The model under review builds one solid part; all positions refer to its coordinate system, in mm. Face numbers are marked on the shaded views. Round coordinates to 2 decimals unless told otherwise and drop trailing zeros. Loops run counter-clockwise (first coordinate to the right, second up) from the corner with the lowest first, then second, coordinate; pieces in that order, holes last. Notation, with made-up numbers: (-36.5, 14.25) -> (21.5, 14.25) arc R21 cw to (21.5, 42.25) -> close; hole circle Ø2 at (27.25, 41). An arc over 180 degrees is marked (long way). Write each question's results on one line, items separated by ' | '. Start each with the question number.
Item 1: We need section C-C (z = 2). Give the boundary of the cut face in (x, y), and give its area (3 significant figures).
Item 2: Mouldability with a two-part tool opening along X and no side actions: class the marked faces 1, 2 and 3 as pulls with the +X half, pulls with the -X half, needs draft (parallel to the pull), parting line crosses it, or undercut.
Item 3: Clearance check with flat-ended pins moving along their axes: pin 1 Ø4 at (x, z) = (52, 6) entering from +Y; pin 2 Ø5 at (y, z) = (24, 7) entering from +X; pin 3 Ø5 at (y, z) = (-45.5, 11.5) entering from -X; pin 4 Ø1 at (x, y) = (30, 16) entering from -Z. State where each tip first meets the part, or that it passes through.
Item 4: For L1, parallel to Y at x = 0, z = 3.5; L2, parallel to Z at x = 25.5, y = -18; L3, parallel to X at y = -19.5, z = 6.75, list the stretches that pass through material, from the lowest coordinate up. Write a range as from..to.
Item 5: We need section A-A (y = 0). Give the boundary of the cut face in (x, z).
Item 6: We need section D-D (y = 37.25). Give the boundary of the cut face in (x, z), and give its area (3 significant figures).
Item 7: We need section B-B (x = -72.5). Give the boundary of the cut face in (y, z), and give its area (3 significant figures).
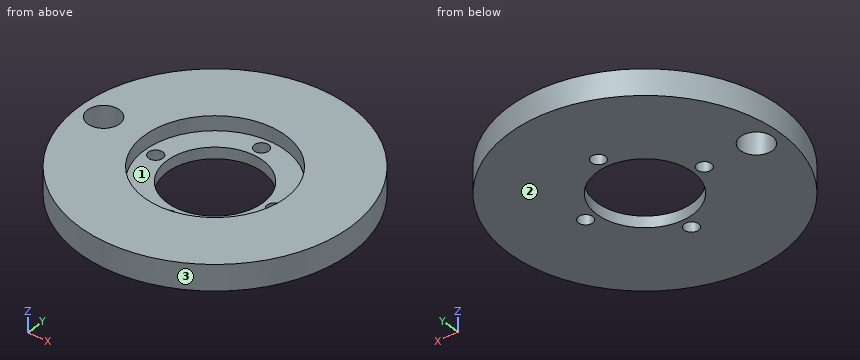
from build123d import *

# Parameters (mm, degrees)
F0_R     = 85
F0_R_2   = 4.5
F0_R_3   = 10
F0_R_4   = 30
F1_DEPTH = 16
F2_R     = 44.25
F2_R_2   = 4.5
F2_R_3   = 30
F3_DEPTH = 9


with BuildPart() as f1:
    # F0 (on Top) → F1 (new body)
    with BuildSketch(Plane.XY):
        Circle(F0_R)
        with Locations((0, -37.25)):
            Circle(F0_R_2, mode=Mode.SUBTRACT)
        with Locations((-70, 0)):
            Circle(F0_R_3, mode=Mode.SUBTRACT)
        with Locations((-37.25, 0)):
            Circle(F0_R_2, mode=Mode.SUBTRACT)
        Circle(F0_R_4, mode=Mode.SUBTRACT)
        with Locations((37.25, 0)):
            Circle(F0_R_2, mode=Mode.SUBTRACT)
        with Locations((0, 37.25)):
            Circle(F0_R_2, mode=Mode.SUBTRACT)
    extrude(amount=F1_DEPTH)

    # F2 (on face) → F3 (cut)
    with BuildSketch(Plane.XY.offset(16)):
        Circle(F2_R)
        with Locations((0, -37.25)):
            Circle(F2_R_2, mode=Mode.SUBTRACT)
        with Locations((-37.25, 0)):
            Circle(F2_R_2, mode=Mode.SUBTRACT)
        Circle(F2_R_3, mode=Mode.SUBTRACT)
        with Locations((37.25, 0)):
            Circle(F2_R_2, mode=Mode.SUBTRACT)
        with Locations((0, 37.25)):
            Circle(F2_R_2, mode=Mode.SUBTRACT)
    extrude(amount=-F3_DEPTH, mode=Mode.SUBTRACT)


solid = f1.part
Here are the results:
1) outline: circle Ø170 at (0, 0); hole circle Ø20 at (-70, 0); hole circle Ø9 at (-37.25, 0); hole circle Ø60 at (0, 0); hole circle Ø9 at (0, -37.25); hole circle Ø9 at (0, 37.25); hole circle Ø9 at (37.25, 0) | area: 19,300 mm2
2) face 1: undercut | face 2: needs draft | face 3: parting line crosses it
3) pin 1: stops at y = 68.74 | pin 2: stops at x = 82.24 | pin 3: stops at x = -73.32 | pin 4: stops at z = 0
4) L1: y = -85..-41.75, -32.75..-30, 30..32.75, 41.75..85 | L2: z = 0..7 | L3: x = -82.73..-22.8, 22.8..82.73
5) outline: (-85, 0) -> (-80, 0) -> (-80, 16) -> (-85, 16) -> close; (-60, 0) -> (-41.75, 0) -> (-41.75, 7) -> (-44.25, 7) -> (-44.25, 16) -> (-60, 16) -> close; (-32.75, 0) -> (-30, 0) -> (-30, 7) -> (-32.75, 7) -> close; (30, 0) -> (32.75, 0) -> (32.75, 7) -> (30, 7) -> close; (41.75, 0) -> (85, 0) -> (85, 16) -> (44.25, 16) -> (44.25, 7) -> (41.75, 7) -> close
6) outline: (-76.4, 0) -> (-4.5, 0) -> (-4.5, 7) -> (-23.89, 7) -> (-23.89, 16) -> (-76.4, 16) -> close; (4.5, 0) -> (76.4, 0) -> (76.4, 16) -> (23.89, 16) -> (23.89, 7) -> (4.5, 7) -> close | area: 1,950 mm2
7) outline: (-44.37, 0) -> (-9.68, 0) -> (-9.68, 16) -> (-44.37, 16) -> close; (9.68, 0) -> (44.37, 0) -> (44.37, 16) -> (9.68, 16) -> close | area: 1,110 mm2
